```python
from build123d import *

# Parameters (mm, degrees)
SKETCH_R        = 25
PAD_DEPTH       = 10
SKETCH001_W     = 20
SKETCH001_H     = 15
PAD001_DEPTH    = 12
SKETCH002_R     = 2.7
POCKET_DEPTH    = 10
SKETCH003_W     = 4.1
SKETCH003_H     = 7.2
POCKET001_DEPTH = 12
SKETCH004_R     = 2.2
POCKET002_DEPTH = 30
FILLET_R        = 5
FILLET001_R     = 5
FILLET002_R     = 5
FILLET003_R     = 5
SKETCH005_R     = 5
PAD002_DEPTH    = 10
SKETCH006_W     = 3.9
SKETCH006_H     = 10
PAD003_DEPTH    = 10
SKETCH007_R     = 2.2
POCKET003_DEPTH = 4
SKETCH008_R     = 8.1
SKETCH008_R_2   = 5
PAD004_DEPTH    = 5
FILLET004_R     = 5
FILLET005_R     = 4.95
CHAMFER_SIZE    = 2
CHAMFER001_SIZE = 2


with BuildPart() as part:
    # Sketch → Pad (new body)
    with BuildSketch(Plane.XY):
        Circle(SKETCH_R)
    extrude(amount=PAD_DEPTH)

    # Sketch001 (on Face3 of Pad) → Pad001 (join)
    with BuildSketch(Plane.XY.offset(10)):
        Rectangle(SKETCH001_W, SKETCH001_H)
    extrude(amount=PAD001_DEPTH)

    # Sketch002 (on Face8 of Pad001) → Pocket (cut)
    with BuildSketch(Plane.XY.offset(22)):
        Circle(SKETCH002_R)
    extrude(amount=-POCKET_DEPTH, mode=Mode.SUBTRACT)

    # Sketch003 (on Face8 of Pocket) → Pocket001 (cut)
    with BuildSketch(Plane.XY.offset(22)):
        with Locations((-6.35, 0)):
            Rectangle(SKETCH003_W, SKETCH003_H)
        with Locations((6.35, 0)):
            Rectangle(SKETCH003_W, SKETCH003_H)
    extrude(amount=-POCKET001_DEPTH, mode=Mode.SUBTRACT)

    # Sketch004 (on Face6 of Pocket001) → Pocket002 (cut)
    with BuildSketch(Plane.YZ.offset(10)):
        with Locations((0, 15)):
            Circle(SKETCH004_R)
    extrude(amount=-POCKET002_DEPTH, mode=Mode.SUBTRACT)

    # Fillet
    fillet_edges = [part.edges().sort_by_distance(p)[0] for p in [
        (-10, -7.5, 16),
    ]]
    fillet(fillet_edges, radius=FILLET_R)

    # Fillet001
    fillet001_edges = [part.edges().sort_by_distance(p)[0] for p in [
        (-10, 7.5, 16),
    ]]
    fillet(fillet001_edges, radius=FILLET001_R)

    # Fillet002
    fillet002_edges = [part.edges().sort_by_distance(p)[0] for p in [
        (10, 7.5, 16),
    ]]
    fillet(fillet002_edges, radius=FILLET002_R)

    # Fillet003
    fillet003_edges = [part.edges().sort_by_distance(p)[0] for p in [
        (10, -7.5, 16),
    ]]
    fillet(fillet003_edges, radius=FILLET003_R)

    # Sketch005 (on Face1 of Fillet003) → Pad002 (join)
    with BuildSketch(Plane.XY.offset(10)):
        with BuildLine():
            Line((-7, 36), (-7, -36))
            ThreePointArc((-7, -36), (-7.103731, -44.222064), (0, -48.363333))
            ThreePointArc((0, -48.363333), (7.103731, -44.222064), (7, -36))
            Line((7, 36), (7, -36))
            ThreePointArc((7, 36), (7.103731, 44.222064), (0, 48.363333))
            ThreePointArc((0, 48.363333), (-7.103731, 44.222064), (-7, 36))
        make_face()
        with Locations((0, -40.2)):
            Circle(SKETCH005_R, mode=Mode.SUBTRACT)
        with Locations((0, 40.2)):
            Circle(SKETCH005_R, mode=Mode.SUBTRACT)
    extrude(amount=-PAD002_DEPTH)

    # Sketch006 (on Face13 of Pad002) → Pad003 (join)
    with BuildSketch(Plane.XY.offset(10)):
        with Locations((-18.95, 0)):
            Rectangle(SKETCH006_W, SKETCH006_H)
    extrude(amount=PAD003_DEPTH)

    # Sketch007 (on Face32 of Pad003) → Pocket003 (cut)
    with BuildSketch(Plane(origin=(-20.9, 0, 0), x_dir=(0, -1, 0), z_dir=(-1, 0, 0))):
        with Locations((0, 15)):
            Circle(SKETCH007_R)
    extrude(amount=-POCKET003_DEPTH, mode=Mode.SUBTRACT)

    # Sketch008 (on Face18 of Pocket003) → Pad004 (join)
    with BuildSketch(Plane.XY.offset(10)):
        with Locations((0, 40.2)):
            Circle(SKETCH008_R)
        with Locations((0, 40.2)):
            Circle(SKETCH008_R_2, mode=Mode.SUBTRACT)
        with Locations((0, -40.2)):
            Circle(SKETCH008_R)
        with Locations((0, -40.2)):
            Circle(SKETCH008_R_2, mode=Mode.SUBTRACT)
    extrude(amount=PAD004_DEPTH)

    # Fillet004
    fillet004_edges = [part.edges().sort_by_distance(p)[0] for p in [
        (-18.95, 5, 20),
    ]]
    fillet(fillet004_edges, radius=FILLET004_R)

    # Fillet005
    fillet005_edges = [part.edges().sort_by_distance(p)[0] for p in [
        (-18.95, -5, 20),
    ]]
    fillet(fillet005_edges, radius=FILLET005_R)

    # Chamfer
    chamfer_edges = [part.edges().sort_by_distance(p)[0] for p in [
        (-5, 40.2, 15),
    ]]
    chamfer(chamfer_edges, length=CHAMFER_SIZE)

    # Chamfer001
    chamfer001_edges = [part.edges().sort_by_distance(p)[0] for p in [
        (-5, -40.2, 15),
    ]]
    chamfer(chamfer001_edges, length=CHAMFER001_SIZE)


solid = part.part
```
Model file for the job. Use its own axes, mm. A direction names the side the tool comes from. Give positions to 0.01 mm unless a question says otherwise; leave off trailing zeros. Loops run counter-clockwise (first coordinate to the right, second up) from the corner with the lowest first, then second, coordinate; pieces in that order, holes last. Notation, with made-up numbers: (51, 44) -> (84, 44) arc R17 ccw to (84, 55) -> close; hole circle Ø1 at (42.25, 41). An arc over 180 degrees is marked (long way). Use CSV: the item, a comma, the result in double quotes. Start each with the question number.
1) Tool access for faces 4 (the cylindrical face through (-19, 4, 18)), 5 (the flat face through (-6, 3.6, 16)), 6 (the flat face through (-10, 1.1, 17.2)), 7 (the flat face through (0, 7.5, 16)): list every direction of +Z, -Z, +X, -X, +Y, -Y with a clear straight run to the whole face (end or side of a thin tool).
2) Slice it at B-B on y = 40.2. Give the cut face in (x, z).
3) Slice it at D-D on x = 15. Give the cut face in (y, z), plus the area to 3 significant figures.
4) Wall check: line 1 (Z direction, x = -9.5, y = 0); line 2 (Y direction, x = 6, z = 10.75); line 3 (Z direction, x = -16, y = 9). Give the ranges that are in metal, low to high.
5) Slice it at C-C on z = 3.75. Give the cut face in (x, y).
6) Mould opens along Z. For faces 1 (the cylindrical face through (-18.977, 2.198, 15.097)), 2 (the cylindrical face through (-18.9, -3.5, 18.6)), 3 (the flat face through (10, 1.1, 17.2)) say: released by +Z, released by -Z, zero draft, split by the parting line, or undercut.
7) Flat gauge pins, fed straight in: pin 1 Ø3 at (y, z) = (-30, 3) entering from +X; pin 2 Ø7 at (y, z) = (0, 15) entering from +X; pin 3 Ø10 at (x, z) = (14, 14.5) entering from -Y; pin 4 Ø3.5 at (x, y) = (-7, 0) entering from +Z. Where does each tip first touch, or does it go through?
8) Slice it at A-A on z = 11. Give the cut face in (x, y), plus the area to 3 significant figures.
Computed values:
1,face 4,"+Z, -X, +Y"
1,face 5,"+Z"
1,face 6,"+Z, +Y, -Y"
1,face 7,"+Z, +X, -X"
2,outline,"(-8.16, 0) -> (-5, 0) -> (-5, 13) -> (-7, 15) -> (-8.1, 15) -> (-8.1, 10) -> (-8.16, 10) -> close; (5, 0) -> (8.16, 0) -> (8.16, 10) -> (8.1, 10) -> (8.1, 15) -> (7, 15) -> (5, 13) -> close"
3,outline,"(-20, 0) -> (20, 0) -> (20, 10) -> (-20, 10) -> close"
3,area,"400 mm^2"
4,line 1,"z = 0 to 12.8, 17.2 to 22"
4,line 2,"y = -45.64 to -34.76, -7.4 to -3.6, 3.6 to 7.4, 34.76 to 45.64"
4,line 3,"z = 0 to 10"
5,outline,"(-7, -36) arc R8.16 ccw to (0, -48.36) arc R8.16 ccw to (7, -36) -> (7, -24) arc R25 ccw to (7, 24) -> (7, 36) arc R8.16 ccw to (0, 48.36) arc R8.16 ccw to (-7, 36) -> (-7, 24) arc R25 ccw to (-7, -24) -> close; hole circle Ø10 at (0, -40.2); hole circle Ø10 at (0, 40.2)"
6,face 1,"undercut"
6,face 2,"released by +Z"
6,face 3,"zero draft"
7,pin 1,"stops at x = 7"
7,pin 2,"stops at x = 10"
7,pin 3,"stops at y = -22.03"
7,pin 4,"stops at z = 22"
8,outline,"(-20.9, -5) -> (-17, -5) -> (-17, 5) -> (-20.9, 5) -> close; (-10, -2.5) arc R5 ccw to (-5, -7.5) -> (5, -7.5) arc R5 ccw to (10, -2.5) -> (10, 2.5) arc R5 ccw to (5, 7.5) -> (-5, 7.5) arc R5 ccw to (-10, 2.5) -> close; circle Ø16.2 at (0, -40.2); circle Ø16.2 at (0, 40.2); hole (-8.4, -3.6) -> (-4.3, -3.6) -> (-4.3, 3.6) -> (-8.4, 3.6) -> close; hole circle Ø10 at (0, -40.2); hole circle Ø10 at (0, 40.2); hole (4.3, -3.6) -> (8.4, -3.6) -> (8.4, 3.6) -> (4.3, 3.6) -> close"
8,area,"514 mm^2"
